from build123d import *

# Parameters (mm, degrees)
SKETCH_R        = 4.225
PAD_DEPTH       = 8
SKETCH001_R     = 7
PAD001_DEPTH    = 1
SKETCH002_R     = 11.25
PAD002_DEPTH    = 8
SKETCH003_R     = 2
POCKET_DEPTH    = 17.001
SKETCH004_R     = 3.25
POCKET001_DEPTH = 3


with BuildPart() as part:
    # Sketch → Pad (new body)
    with BuildSketch(Plane.XY):
        Circle(SKETCH_R)
    extrude(amount=PAD_DEPTH)

    # Sketch001 → Pad001 (join)
    with BuildSketch(Plane.XY):
        Circle(SKETCH001_R)
    extrude(amount=-PAD001_DEPTH)

    # Sketch002 (on Face3 of Pad001) → Pad002 (join)
    with BuildSketch(Plane(origin=(0, 0, -1), x_dir=(1, 0, 0), z_dir=(0, 0, -1))):
        Circle(SKETCH002_R)
    extrude(amount=PAD002_DEPTH)

    # Sketch003 (on Face3 of Pad002) → Pocket (cut, through all)
    with BuildSketch(Plane(origin=(0, 0, -9), x_dir=(1, 0, 0), z_dir=(0, 0, -1))):
        Circle(SKETCH003_R)
    extrude(amount=-POCKET_DEPTH, mode=Mode.SUBTRACT)

    # Sketch004 (on Face3 of Pocket) → Pocket001 (cut)
    with BuildSketch(Plane(origin=(0, 0, -9), x_dir=(1, 0, 0), z_dir=(0, 0, -1))):
        Circle(SKETCH004_R)
    extrude(amount=-POCKET001_DEPTH, mode=Mode.SUBTRACT)


solid = part.part
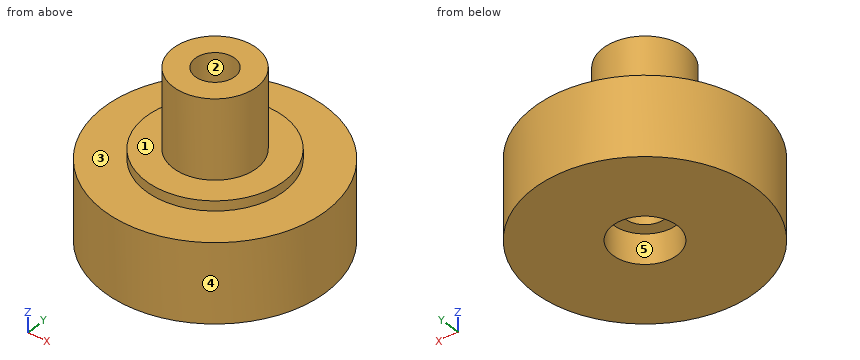
The listing builds one solid part. Answer for the finished solid, in the listing's coordinates (mm). Face numbers are marked on the shaded views. A direction names the side the tool comes from. Coordinates: 2 decimals unless noted, no trailing zeros. Write each loop counter-clockwise with the first axis right and the second up, starting at its lowest first coordinate (ties: lowest second). Pieces come first, ordered by that corner, then holes. Notation, with made-up numbers: (8.5, 38.25) - (26.5, 38.25) arc R18 cw to (26.5, 72.25) - close; hole circle Ø2 at (33.5, -19.75). An arc over 180 degrees is marked (long way). Answer as CSV lines item,"result".
1. Given P1, Ø1, axis at y = -5, z = -5, coming from the -X side; P2, Ø2, axis at y = -6, z = 2.5, coming from the -X side; P3, Ø5, axis at x = 9, y = -1.5, coming from the +Z side, each flat-ended and moving along its own axis, determine where each tip first touches the part or whether it passes through.
Computed values:
P1,"stops at x = -10.31"
P2,"passes through"
P3,"stops at z = 0"
2. Find section A-A (x = 0). Give the vertices of the cut face in (y, z) (3 decimals).
Computed values:
outline,"(-11.25, -9) - (-3.25, -9) - (-3.25, -6) - (-2, -6) - (-2, 8) - (-4.225, 8) - (-4.225, 0) - (-7, 0) - (-7, -1) - (-11.25, -1) - close; (2, -6) - (3.25, -6) - (3.25, -9) - (11.25, -9) - (11.25, -1) - (7, -1) - (7, 0) - (4.225, 0) - (4.225, 8) - (2, 8) - close"
3. A tool of negligible diameter and unlimited length cuts with its end or side. For the marked faces 1 and 2, from which of +Z, -Z, +X, -X, +Y, -Y can it reach the whole face along a straight path? Write none if from no direction.
Computed values:
face 1,"+Z"
face 2,"+Z, -Z"
4. Determine the mould class of the marked faces 3, 4 and 5 for opening direction X: +X half, -X half, draft (parallel to the pull), parting line (faces both ways), or undercut.
Computed values:
face 3,"draft"
face 4,"parting line"
face 5,"undercut"
5. Straight lines are drawn through the part: line 1 (Y direction, x = 0, z = -8.1); line 2 (Y direction, x = 0, z = -1.25); line 3 (Z direction, x = 1, y = 5.25). For each, find the intervals that lie inside material, in ascending order. Write a range as [from, to].
Computed values:
line 1,"y = [-11.25, -3.25], [3.25, 11.25]"
line 2,"y = [-11.25, -2], [2, 11.25]"
line 3,"z = [-9, 0]"
6. Find section D-D (y = -6.5). Give the vertices of the cut face in (x, z).
Computed values:
outline,"(-9.18, -9) - (9.18, -9) - (9.18, -1) - (2.6, -1) - (2.6, 0) - (-2.6, 0) - (-2.6, -1) - (-9.18, -1) - close"
7. Find section C-C (z = -5.25). Give the vertices of the cut face in (x, y), plus the area to 3 significant figures.
Computed values:
outline,"circle Ø22.5 at (0, 0); hole circle Ø4 at (0, 0)"
area,"385 mm²"
